Source: CAD feature listing. Evaluate the final solid. Frame: model axes, mm. A direction names the side the tool comes from. Give positions to 0.01 mm unless a question says otherwise; leave off trailing zeros. Order: outer loops, then holes, each group sorted by start corner. A loop starts at its lowest first (then second) coordinate and runs counter-clockwise, first axis right, second up.
Autodesk Fusion 360 part; units mm, degrees
sketch "草图1" plane through (0, 0, 0) normal (0, 1, 0) x (1, 0, 0)
  line L0 (0, 0) -> (44.6777, 0)
  line L1 (44.6777, 0) -> (59.3388, -14.6612)
  arc A0 (41.6612, -32.3388) -> (59.3388, -14.6612) centre (50.5, -23.5) ccw
  line L2 (41.6612, -32.3388) -> (30.3223, -21)
  line L3 (30.3223, -21) -> (-16.5083, -15)
  arc A1 (-20, -11.0324) -> (-16.5083, -15) centre (-16, -11.0324) ccw
  line L4 (-20, -11.0324) -> (-20, -5)
  line L5 (-20, -5) -> (0, -5)
  line L6 (0, -5) -> (0, 0)
  circle A2 centre (35, -7) radius 2.5
  dimension "d1" = 5
  dimension "d2" = 20
  dimension "d3" = 4
  dimension "d4" = 135
  dimension "d5" = 35
  dimension "d6" = 12.5
  dimension "d7" = 23.5
  dimension "d8" = 70.5
  dimension "d9" = 5
  dimension "d10" = 7
  dimension "d11" = 21
  dimension "d12" = 10
extrude "拉伸1" add sketch "草图1" along normal blind 35
sketch "草图2" plane through (0, 0, 0) normal (0, 0, 1) x (1, 0, 0)
  line L0 (-20, 0) -> (-20, 35)
  line L1 (-20, 35) -> (16, 35)
  line L2 (16, 35) -> (21, 30)
  line L3 (21, 30) -> (105, 30)
  line L4 (105, 30) -> (105, 5)
  line L5 (105, 5) -> (21, 5)
  line L6 (21, 5) -> (16, 0)
  line L7 (16, 0) -> (-20, 0)
  line L8 (-55, 0) -> (65, 0) construction
  line L9 (-20, 17.5) -> (-60, 17.5) construction
  dimension "d15" = 20
  dimension "d16" = 35
  dimension "d17" = 36
  dimension "d18" = 135
  dimension "d19" = 135
  dimension "d20" = 25
  dimension "d21" = 125
extrude "拉伸2" cut sketch "草图2" along normal blind 85 keep common part
sketch "草图3" plane through (4.6612, 0, -4.6612) normal (-0.7071, 0, 0.7071) x (0, -1, 0)
  line L0 (-30, 52.3259) -> (-30, 36.2904)
  line L1 (-30, 36.2904) -> (-5, 36.2904)
  line L2 (-5, 36.2904) -> (-5, 52.3259)
  line L3 (-5, 52.3259) -> (-30, 52.3259)
  line L4 (-17.5, 36.2904) -> (-17.5, 72) construction
  line L5 (-19.5, 39.8259) -> (-15.5, 39.8259)
  line L6 (-12.5, 39.8259) -> (-12.5, 64.8259)
  line L7 (-12.5, 64.8259) -> (-22.5, 64.8259)
  line L8 (-22.5, 64.8259) -> (-22.5, 42.8259)
  arc A0 (-15.5, 39.8259) -> (-12.5, 42.8259) centre (-12.5, 39.8259) ccw
  arc A1 (-22.5, 42.8259) -> (-19.5, 39.8259) centre (-22.5, 39.8259) ccw
  dimension "d24" = 6
  dimension "d25" = 10
  dimension "d26" = 12.5
  dimension "d27" = 25
extrude "拉伸3" cut sketch "草图3" against normal blind 61 contours L3 L6 L7 L8 | L3 L5 L6 L8 A0 A1
sketch "草图4" plane through (0, 30, 0) normal (0, 1, 0) x (-1, 0, 0)
  line L0 (-21, 19.8056) -> (-30.3223, 21)
  line L1 (-30.3223, 21) -> (-41.6612, 32.3388)
  arc A0 (-41.6612, 32.3388) -> (-59.3388, 14.6612) centre (-50.5, 23.5) ccw
  line L2 (-59.3388, 14.6612) -> (-44.6777, 0)
  line L3 (-44.6777, 0) -> (-21, 0)
  line L4 (-21, 0) -> (-21, 19.8056)
  circle A1 centre (-35, 7) radius 2.5
  circle A2 centre (-50.5, 23.5) radius 3.5
  dimension "d30" = 7
extrude "拉伸4" cut sketch "草图4" against normal blind 15 contours A2
sketch "草图5" plane through (0, 5, 0) normal (0, -1, 0) x (1, 0, 0)
  line L0 (30.3223, 21) -> (21, 19.8056)
  line L1 (21, 19.8056) -> (21, 0)
  line L2 (21, 0) -> (44.6777, 0)
  line L3 (44.6777, 0) -> (59.3388, 14.6612)
  arc A0 (59.3388, 14.6612) -> (41.6612, 32.3388) centre (50.5, 23.5) ccw
  line L4 (41.6612, 32.3388) -> (30.3223, 21)
  circle A1 centre (35, 7) radius 2.5
hole "孔1" at (50.5, 5, 23.5) direction (0, 1, 0) diameter 6 depth 13 tip angle 180
thread "螺纹1" thread offset 0 thread length 10
sketch "草图6" plane through (0, 0, 0) normal (0, 0, -1) x (1, 0, 0)
  line L0 (16, -35) -> (21, -30)
  line L1 (21, -30) -> (44.6777, -30)
  line L2 (44.6777, -30) -> (44.6777, -5)
  line L3 (44.6777, -5) -> (21, -5)
  line L4 (21, -5) -> (16, 0)
  line L5 (16, 0) -> (0, 0)
  line L6 (0, 0) -> (0, -35)
  line L7 (0, -35) -> (16, -35)
  circle A0 centre (7, -17.5) radius 4.5
  dimension "d38" = 7
  dimension "d39" = 9
  dimension "d40" = 17.5
extrude "拉伸5" cut sketch "草图6" against normal blind 5 contours A0
sketch "草图7" plane through (0, 0, 5) normal (0, 0, -1) x (1, 0, 0)
  circle A0 centre (7, -17.5) radius 4.5
  circle A1 centre (7, -17.5) radius 3
  dimension "d43" = 6
extrude "拉伸6" cut sketch "草图7" against normal blind 92 contours A1
thread "螺纹2" thread offset 0 thread length 10
equation "d26 = 25 mm - 12.5 mm"
1) Material intervals for L1, parallel to Y at x = 7, z = 9; L2, parallel to X at y = 11, z = 12; L3, parallel to Z at x = 35.5, y = 29.5, sorted ascending.
Report:
L1: y = 0 to 14.5, 20.5 to 35
L2: x = -19.88 to 40.65, 48 to 56.68
L3: z = 0 to 4.55, 9.45 to 26.18
2) Section query C-C, the plane x = 7. Return the cut outline in (y, z).
Report:
outline: (0, 0) - (13, 0) - (13, 5) - (14.5, 5) - (14.5, 18.01) - (0, 18.01) - close; (20.5, 5) - (22, 5) - (22, 0) - (35, 0) - (35, 18.01) - (20.5, 18.01) - close
3) Section query A-A, the plane y = 24.5. Return the cut outline in (x, z).
Report:
outline: (-20, 5) - (0, 5) - (0, 0) - (44.68, 0) - (48.92, 4.24) - (31.24, 21.92) - (30.32, 21) - (-16.51, 15) arc R4 ccw to (-20, 11.03) - close; (34.4, 25.08) - (52.08, 7.4) - (59.34, 14.66) arc R12.5 ccw to (41.66, 32.34) - close; hole circle Ø5 at (35, 7); hole circle Ø7 at (50.5, 23.5)
4) Draft query along X for faces 6 (the cylindrical face through (47.526, 8.802, 23.891)), 7 (the flat face through (32.29, 17.32, 22.97)), 8 (the cylindrical face through (59.531, 26.197, 32.142)), 9 (the flat face through (49, 12.5, 27)). Return one class per face: +X half, -X half, draft (parallel to the pull), parting line (faces both ways), or undercut.
Report:
face 6: undercut
face 7: -X half
face 8: parting line
face 9: draft
5) Reachability of faces 1 (the flat face through (42, 30, 18)), 2 (the flat face through (41.54, 17.53, 14.78)), 3 (the flat face through (10, 16, 5)), 4 (the flat face through (2, 35, 9)), 5 (the flat face through (-10, 17, 5)) from +Z, -Z, +X, -X, +Y, -Y: full face, straight path, thin tool, end or side. Return the list, or none.
Report:
face 1: +Z, -Z, +X, +Y
face 2: +Z, +X
face 3: -Z
face 4: +Z, -Z, +X, -X, +Y
face 5: -Z, -X, +Y, -Y
6) Section query B-B, the plane y = 17.5. Return the cut outline in (x, z), and give its area (3 significant figures).
Report:
outline: (-20, 5) - (0, 5) - (0, 0) - (2.5, 0) - (2.5, 5) - (4, 5) - (4, 17.63) - (-16.51, 15) arc R4 ccw to (-20, 11.03) - close; (10, 5) - (11.5, 5) - (11.5, 0) - (44.68, 0) - (50.5, 5.82) - (32.82, 23.5) - (30.32, 21) - (10, 18.4) - close; hole circle Ø5 at (35, 7)
area: 947 mm2
7) Pin query (flat end, axial travel): pin 1 (8.5 mm diameter, centred on x = 52.5, z = 18, fed in from -Y); pin 2 (8 mm diameter, centred on x = 7, y = 17.5, fed in from -Z); pin 3 (8 mm diameter, centred on x = 35, z = 7, fed in from +Y). Return the tip coordinate at first contact, or that it passes through.
Report:
pin 1: stops at y = 5
pin 2: stops at z = 5
pin 3: stops at y = 30
8) Section query D-D, the plane z = 7. Count the separate pieces of the cut face and the enclosed holes in it, and give its area (3 significant figures).
Report:
separate pieces: 2
enclosed holes: 1
area: 1,950 mm2
